Geometry: final body of the model. Coordinates: model frame, mm. Face numbers are marked on the shaded views. A direction names the side the tool comes from. Give positions to 0.01 mm unless a question says otherwise; leave off trailing zeros. Loops run counter-clockwise (first coordinate to the right, second up) from the corner with the lowest first, then second, coordinate; pieces in that order, holes last.
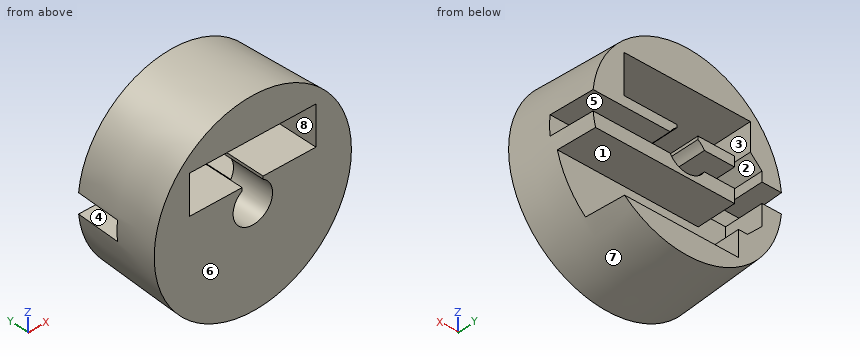
```python
from build123d import *

# Parameters (mm, degrees)
SKETCH_2_R          = 12
SKETCH_1_R          = 12.5
CUT_EXTRUDE_1_DEPTH = 12.0000001
SKETCH_5_W          = 13
SKETCH_5_H          = 6
CUT_EXTRUDE_2_DEPTH = 5
SKETCH_6_W          = 2.476692414
SKETCH_6_H          = 6.83521307
CUT_EXTRUDE_3_DEPTH = 20
CUT_EXTRUDE_4_DEPTH = 5


with BuildPart() as part:
    # 草图2 → 放样1 section 0
    with BuildSketch(Plane(origin=(0, 11, 0), x_dir=(1, 0, 0), z_dir=(0, 1, 0))):
        Circle(SKETCH_2_R)
    # 草图1 → 放样1 section 1
    with BuildSketch(Plane(origin=(0, 0, 0), x_dir=(1, 0, 0), z_dir=(0, 1, 0))):
        Circle(SKETCH_1_R)
    loft()

    # 草图4 → 切除-拉伸1 (cut, through all)
    with BuildSketch(Plane(origin=(0, 0, 0), x_dir=(1, 0, 0), z_dir=(0, 1, 0))):
        with BuildLine():
            Line((-1.352272566, -2.5), (-1.352272566, -2.102702762))
            ThreePointArc((-1.352272566, -2.102702762), (0.025010963, 2.499874887), (1.309931483, -2.12933781))
            Line((1.309931483, -2.12933781), (1.309931483, -2.5))
            Line((1.309931483, -2.5), (8, -2.5))
            Line((8, -2.5), (8, -7.5))
            Line((8, -7.5), (-8, -7.5))
            Line((-8, -7.5), (-8, -2.5))
            Line((-8, -2.5), (-1.352272566, -2.5))
        make_face()
    extrude(amount=CUT_EXTRUDE_1_DEPTH, mode=Mode.SUBTRACT)

    # 草图5 → 切除-拉伸2 (cut)
    with BuildSketch(Plane(origin=(0, 11, 0), x_dir=(1, 0, 0), z_dir=(0, 1, 0))):
        with Locations((0, 5.991032562)):
            Rectangle(SKETCH_5_W, SKETCH_5_H)
        with BuildLine():
            Line((7.947410488, 8.991032562), (6.5, 8.991032562))
            Line((6.5, 8.991032562), (6.5, 2.991032562))
            Line((6.5, 2.991032562), (11.621261731, 2.991032562))
            ThreePointArc((11.621261731, 2.991032562), (10.233925596, 6.266320045), (7.947410488, 8.991032562))
        make_face()
        with BuildLine():
            Line((15.348611284, 8.991032562), (7.947410488, 8.991032562))
            ThreePointArc((7.947410488, 8.991032562), (10.233925596, 6.266320045), (11.621261731, 2.991032562))
            Line((11.621261731, 2.991032562), (15.348611284, 2.991032562))
            Line((15.348611284, 2.991032562), (15.348611284, 8.991032562))
        make_face()
    extrude(amount=-CUT_EXTRUDE_2_DEPTH, mode=Mode.SUBTRACT)

    # 草图6 → 切除-拉伸3 (cut, symmetric)
    with BuildSketch(Plane(origin=(0, 0, 0), x_dir=(0, 0, -1), z_dir=(1, 0, 0))):
        with Locations((0, 8.790545757)):
            Rectangle(SKETCH_6_W, SKETCH_6_H)
    extrude(amount=CUT_EXTRUDE_3_DEPTH, both=True, mode=Mode.SUBTRACT)

    # 草图7 → 切除-拉伸4 (cut)
    with BuildSketch(Plane(origin=(0, 11, 0), x_dir=(1, 0, 0), z_dir=(0, 1, 0))):
        Polygon((-5.998196858, 2.991032562), (-5.998196858, -3.96939498), (-8, -3.96939498), (-9.46939498, -2.5), (-9.46939498, 3.910589128), (-7.645587141, 5.734396966), (-6.5, 5.734396966), align=None)
    extrude(amount=-CUT_EXTRUDE_4_DEPTH, mode=Mode.SUBTRACT)


solid = part.part
```
Q1. Reachability of the marked faces 1, 2, 3 and 4 from +Z, -Z, +X, -X, +Y, -Y: full face, straight path, thin tool, end or side. Return the list, or none.
Q2. Section query C-C, the plane y = 3.75. Return loops of the section in (x, z), and give its area (3 significant figures).
Q3. Section query A-A, the plane x = 0. Return loops of the section in (y, z), and give its area (4 significant figures).
Q4. Section query B-B, the plane y = 9.75. State how many separate pieces and enclosed holes the cut face has, and give its area (3 significant figures).
Q5. Pin query (flat end, axial travel): pin 1 Ø6 at (y, z) = (8.5, 1.5) entering from -X; pin 2 Ø3 at (x, y) = (-5.5, 8) entering from +Z; pin 3 Ø4 at (x, y) = (-7.5, 1.5) entering from -Z. Return the tip coordinate at first contact, or that it passes through.
Q6. Material intervals for probe 1 along Z at (x, y) = (0, 6.5); probe 2 along Z at (x, y) = (-1.5, 6.5); probe 3 along Z at (x, y) = (1.75, 5), sorted ascending.
Q7. Mould query, pull axis Z, two halves, no side actions, for the marked faces 5, 6, 7 and 8. Classes: +Z half, -Z half, draft (parallel to the pull), parting line (faces both ways), or undercut.
Resolved:
1. face 1: +X, +Y
1. face 2: +Y
1. face 3: +Y, -Y
1. face 4: +X, -X, +Y
2. outline: circle Ø24.66 at (0, 0); hole (-8, 2.5) - (-1.35, 2.5) - (-1.35, 2.1) arc R2.5 ccw (long way) to (1.31, 2.13) - (1.31, 2.5) - (8, 2.5) - (8, 7.5) - (-8, 7.5) - close
2. area: 378 mm2
3. outline: (0, -12.5) - (11, -12) - (11, -8.99) - (6, -8.99) - (6, -2.99) - (11, -2.99) - (11, -2.5) - (0, -2.5) - close; (0, 7.5) - (11, 7.5) - (11, 12) - (0, 12.5) - close
3. area: 129.5 mm2
4. separate pieces: 4
4. enclosed holes: 0
4. area: 190 mm2
5. pin 1: stops at x = -12.19
5. pin 2: stops at z = 11.46
5. pin 3: stops at z = -11.15
6. probe 1: z = -12.2 to -8.99, -2.99 to -2.5, 7.5 to 12.2
6. probe 2: z = -12.11 to -8.99, -2.99 to -2, 2 to 2.5, 7.5 to 12.11
6. probe 3: z = -12.15 to -1.79, 1.79 to 2.5, 7.5 to 12.15
7. face 5: undercut
7. face 6: draft
7. face 7: parting line
7. face 8: undercut
